The figure shows three views and two pictorial views of one solid part (mm, origin at its lowest corner). Answer the questions. A direction names the side the tool comes from. Coordinates: 2 decimals unless noted, no trailing zeros. Write each loop counter-clockwise with the first axis right and the second up, starting at its lowest first coordinate (ties: lowest second). Pieces come first, ordered by that corner, then holes. Notation, with made-up numbers: M 41.25,72.5 L 57.25,72.5 A12 cw 57.25,87.5 Z; hole C -31.5,48.25 d4. An arc over 180 degrees is marked long. Write item = value, one per line.
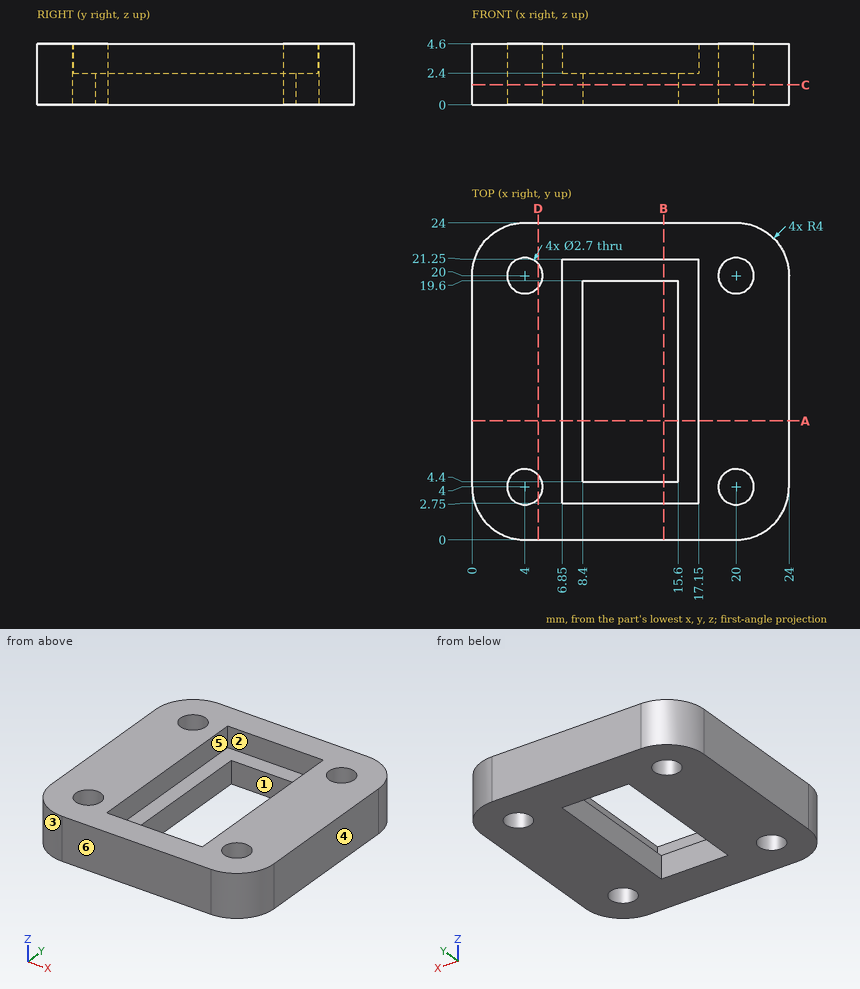
Item 1: For a pull along X with two mould halves and no side action, classify the marked faces 4, 5 and 6 as released by +X, released by -X, zero draft, split by the parting line, or undercut.
Worked answers:
face_4 = released by +X
face_5 = undercut
face_6 = zero draft
Item 2: Find section A-A (y = 9). Determine the outline of the cut face in (x, z), and give its area (3 significant figures).
Worked answers:
outline = M 0,0 L 8.4,0 L 8.4,2.4 L 6.85,2.4 L 6.85,4.6 L 0,4.6 Z; M 15.6,0 L 24,0 L 24,4.6 L 17.15,4.6 L 17.15,2.4 L 15.6,2.4 Z
area = 70.5 mm²
Item 3: Find section C-C (z = 1.5). Determine the outline of the cut face in (x, y), and give its area (3 significant figures).
Worked answers:
outline = M 0,4 A4 ccw 4,0 L 20,0 A4 ccw 24,4 L 24,20 A4 ccw 20,24 L 4,24 A4 ccw 0,20 Z; hole C 4,4 d2.7; hole C 4,20 d2.7; hole M 8.4,4.4 L 15.6,4.4 L 15.6,19.6 L 8.4,19.6 Z; hole C 20,4 d2.7; hole C 20,20 d2.7
area = 430 mm²
Item 4: Find section D-D (x = 5). Determine the outline of the cut face in (y, z), and give its area (3 significant figures).
Worked answers:
outline = M 0,0 L 3.09,0 L 3.09,4.6 L 0,4.6 Z; M 4.91,0 L 19.09,0 L 19.09,4.6 L 4.91,4.6 Z; M 20.91,0 L 24,0 L 24,4.6 L 20.91,4.6 Z
area = 93.7 mm²
Item 5: Consider line 1 along Y through (x, z) = (20, 1.4); line 2 along X through (y, z) = (13.5, 3.4); line 3 along Y through (x, z) = (14, 0.95). Determine where each line is inside the solid, lowest interval first. Write a range as from..to.
Worked answers:
line_1 = 0..2.65, 5.35..18.65, 21.35..24
line_2 = 0..6.85, 17.15..24
line_3 = 0..4.4, 19.6..24
Item 6: Find section B-B (x = 14.5). Determine the outline of the cut face in (y, z), and give its area (3 significant figures).
Worked answers:
outline = M 0,0 L 4.4,0 L 4.4,2.4 L 2.75,2.4 L 2.75,4.6 L 0,4.6 Z; M 19.6,0 L 24,0 L 24,4.6 L 21.25,4.6 L 21.25,2.4 L 19.6,2.4 Z
area = 33.2 mm²
Item 7: Which of the six approach directions +Z, -Z, +X, -X, +Y, -Y give full straight-line access (tool end or side, diameter ignored) to the marked faces 1, 2 and 3?
Worked answers:
face_1 = +Z, -Z
face_2 = +Z
face_3 = +Z, -Z, -X, -Y
